Input: dimensioned drawing with shaded views. Units: mm. Origin: part minimum x, y, z. Coordinates: 2 decimals unless noted, no trailing zeros. Order: outer loops, then holes, each group sorted by start corner. A loop starts at its lowest first (then second) coordinate and runs counter-clockwise, first axis right, second up.
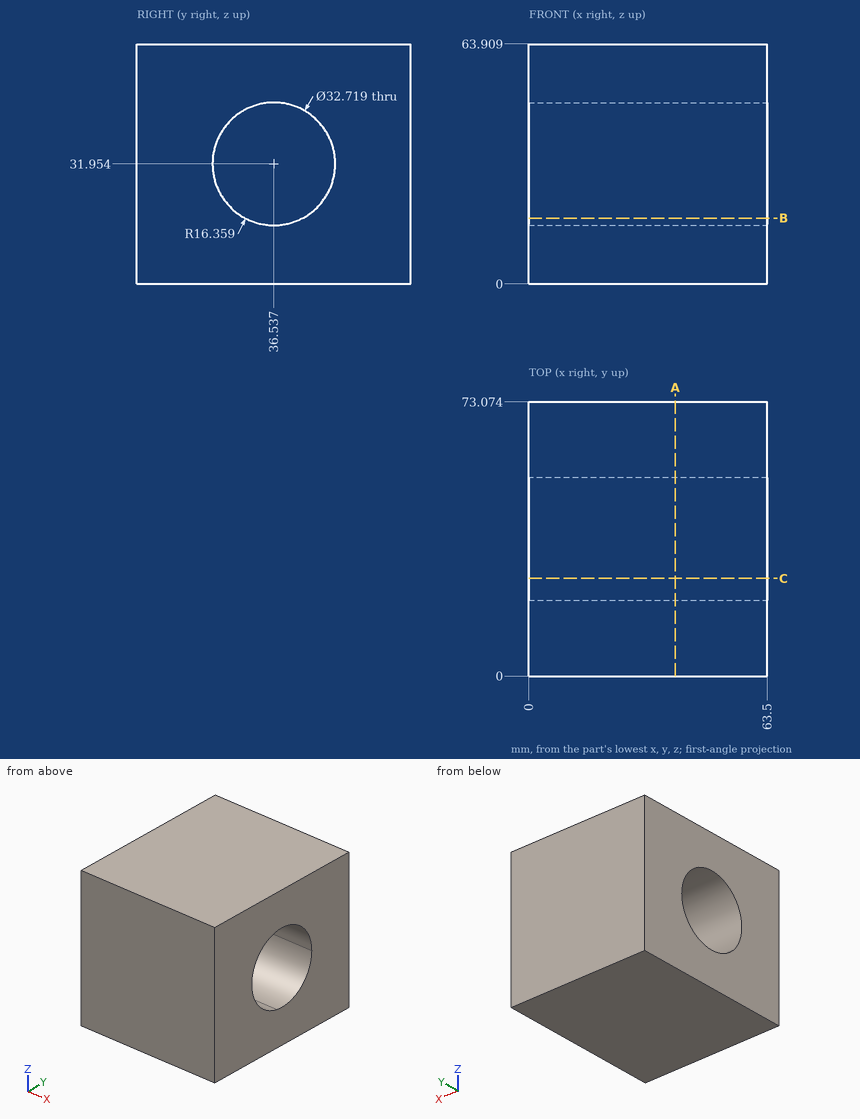
1. Ray query, line 1 (Y direction, x = 13.5, z = 22.5) (1 decimal); line 2 (Y direction, x = 23.5, z = 47) (1 decimal); line 3 (Z direction, x = 32, y = 23.5) (1 decimal). Return the intervals inside material, ascending.
Findings:
line 1: y = 0 to 23.2, 49.9 to 73.1
line 2: y = 0 to 30.1, 43 to 73.1
line 3: z = 0 to 22.1, 41.8 to 63.9
2. Section query A-A on x = 39. Return loops of the section in (y, z) (1 decimal), plus the area to 3 significant figures.
Findings:
outline: (0, 0) - (73.1, 0) - (73.1, 63.9) - (0, 63.9) - close; hole (24.9, 20.5) arc R16.4 ccw to (33.9, 15.8) arc R16.4 ccw (long way) to start
area: 3,830 mm2
3. Section query C-C on y = 26. Return loops of the section in (x, z), plus the area to 3 significant figures.
Findings:
outline: (0, 0) - (63.5, 0) - (63.5, 19.44) - (0, 19.44) - close; (0, 44.47) - (63.5, 44.47) - (63.5, 63.91) - (0, 63.91) - close
area: 2,470 mm2
4. Section query B-B on z = 17.5. Return loops of the section in (x, y) (1 decimal), plus the area to 3 significant figures.
Findings:
outline: (0, 0) - (63.5, 0) - (63.5, 28.9) - (0, 28.9) - close; (0, 44.2) - (63.5, 44.2) - (63.5, 73.1) - (0, 73.1) - close
area: 3,670 mm2
